```python
from build123d import *

# Parameters (mm, degrees)
SKETCH_1_R          = 28.5
SKETCH_1_W          = 5
SKETCH_1_H          = 57
EXTRUDE_1_DEPTH     = 5
SKETCH_2_R          = 1.6
SKETCH_2_R_2        = 20
EXTRUDE_2_DEPTH     = 5
FILLET_1_R          = 10
FILLET_2_R          = 5
SKETCH_3_R          = 1.6
SKETCH_3_R_2        = 7.5
CUT_EXTRUDE_1_DEPTH = 5


with BuildPart() as part:
    # 草图1 → 凸台-拉伸1 (new body)
    with BuildSketch(Plane(origin=(0, 0, 0), x_dir=(1, 0, 0), z_dir=(0, 1, 0))):
        with BuildLine():
            ThreePointArc((0, -28.5), (-28.5, 0), (0, 28.5))
            Line((0, 28.5), (-35, 28.5))
            Line((-35, 28.5), (-35, -28.5))
            Line((-35, -28.5), (0, -28.5))
        make_face()
        Circle(SKETCH_1_R)
        with Locations((-37.5, 0)):
            Rectangle(SKETCH_1_W, SKETCH_1_H)
    extrude(amount=EXTRUDE_1_DEPTH)

    # 草图2 → 凸台-拉伸2 (add)
    with BuildSketch(Plane.ZY.offset(40)):
        with BuildLine():
            Line((28.5, 0), (28.5, 40))
            ThreePointArc((28.5, 40), (0, 68.5), (-28.5, 40))
            Line((-28.5, 40), (-28.5, 0))
            Line((-28.5, 0), (28.5, 0))
        make_face()
        with Locations((12.5, 61.650635095)):
            Circle(SKETCH_2_R, mode=Mode.SUBTRACT)
        with Locations((-12.5, 18.349364905)):
            Circle(SKETCH_2_R, mode=Mode.SUBTRACT)
        with Locations((12.5, 18.349364905)):
            Circle(SKETCH_2_R, mode=Mode.SUBTRACT)
        with Locations((-25, 40)):
            Circle(SKETCH_2_R, mode=Mode.SUBTRACT)
        with Locations((-12.5, 61.650635095)):
            Circle(SKETCH_2_R, mode=Mode.SUBTRACT)
        with Locations((0, 40)):
            Circle(SKETCH_2_R_2, mode=Mode.SUBTRACT)
        with Locations((25, 40)):
            Circle(SKETCH_2_R, mode=Mode.SUBTRACT)
    extrude(amount=-EXTRUDE_2_DEPTH)

    # 圆角1
    fillet_1_edges = [part.edges().sort_by_distance(p)[0] for p in [
        (-40, 0, 0),
    ]]
    fillet(fillet_1_edges, radius=FILLET_1_R)

    # 圆角2
    fillet_2_edges = [part.edges().sort_by_distance(p)[0] for p in [
        (-35, 5, 0),
    ]]
    fillet(fillet_2_edges, radius=FILLET_2_R)

    # 草图3 → 切除-拉伸1 (cut)
    with BuildSketch(Plane(origin=(0, 5, 0), x_dir=(1, 0, 0), z_dir=(0, 1, 0))):
        with Locations((13.5, 0)):
            Circle(SKETCH_3_R)
        with Locations((6.75, -11.691342951)):
            Circle(SKETCH_3_R)
        with Locations((-6.75, -11.691342951)):
            Circle(SKETCH_3_R)
        with Locations((-13.5, 0)):
            Circle(SKETCH_3_R)
        with Locations((-6.75, 11.691342951)):
            Circle(SKETCH_3_R)
        with Locations((6.75, 11.691342951)):
            Circle(SKETCH_3_R)
        Circle(SKETCH_3_R_2)
    extrude(amount=-CUT_EXTRUDE_1_DEPTH, mode=Mode.SUBTRACT)


solid = part.part
```
For this review, take the finished solid that the model builds, in its own axes (mm). A direction names the side the tool comes from. Round coordinates to 2 decimals unless told otherwise and drop trailing zeros. Write each loop counter-clockwise with the first axis right and the second up, starting at its lowest first coordinate (ties: lowest second). Pieces come first, ordered by that corner, then holes. Notation, with made-up numbers: (54.25, -27.75) -> (109.25, -27.75) arc R16 ccw to (109.25, 3.25) -> close; hole circle Ø6 at (80.5, 37.5). An arc over 180 degrees is marked (long way). One line per question, with ' | ' between items. Start each with the question number.
(1) Add section B-B, the plane x = -13.5. Write out the cut boundary in (y, z).
(2) For line 1 along Z through (x, y) = (-6, 3); line 2 along Z through (x, y) = (-6.75, 2.85); line 3 along Y through (x, z) = (-26, 25.5), list the stretches that pass through material, from the lowest coordinate up. Write a range as from..to.
(3) Add section D-D, the plane z = 25. Write out the cut boundary in (x, y).
(4) Insertion check: P1, Ø3, axis at x = -13.5, z = 0, coming from the +Y side; P2, Ø2, axis at x = -31.5, z = 4, coming from the +Y side; P3, Ø8, axis at y = 36.5, z = 20.5, coming from the +X side; P4, Ø2, axis at x = 6, z = -8.5, coming from the +Y side. Each pin has a flat end and moves straight along its axis. Give the tip position at first contact, or say it passes through.
(5) Mouldability with a two-part tool opening along X and no side actions: class faces 1 (the face through (28.493, 2.465, 0.627)), 2 (the face through (6.542, 2.535, -13.278)), 3 (the face through (-8, 0, 0)) as released by +X, released by -X, zero draft, split by the parting line, or undercut.
(6) Add section A-A, the plane z = 0. Write out the cut boundary in (x, y).
(7) Tool access review of faces 4 (the face through (-35, 20, 6)), 5 (the face through (-40, 19, 0)): name each direction out of +Z, -Z, +X, -X, +Y, -Y from which nothing blocks a thin tool from reaching the whole face with its end or side.
(8) Add section C-C, the plane y = 23. Write out the cut boundary in (x, z).
Answer list:
1) outline: (0, -28.5) -> (5, -28.5) -> (5, -1.6) -> (0, -1.6) -> close; (0, 1.6) -> (5, 1.6) -> (5, 28.5) -> (0, 28.5) -> close
2) line 1: -28.5..-13.1, -10.28..-4.5, 4.5..10.28, 13.1..28.5 | line 2: -28.5..-13.29, -10.09..-3.27, 3.27..10.09, 13.29..28.5 | line 3: 0..5
3) outline: (-40, 10) arc R10 ccw to (-30, 0) -> (13.68, 0) -> (13.68, 5) -> (-30, 5) arc R5 cw to (-35, 10) -> (-35, 38.4) -> (-40, 38.4) -> close; (-40, 41.6) -> (-35, 41.6) -> (-35, 53.68) -> (-40, 53.68) -> close
4) P1: through | P2: y = 5.67 | P3: x = -35 | P4: y = 5
5) face 1: released by +X | face 2: undercut | face 3: zero draft
6) outline: (-40, 10) arc R10 ccw to (-30, 0) -> (-15.1, 0) -> (-15.1, 5) -> (-30, 5) arc R5 cw to (-35, 10) -> (-35, 20) -> (-40, 20) -> close; (-40, 60) -> (-35, 60) -> (-35, 68.5) -> (-40, 68.5) -> close; (-11.9, 0) -> (-7.5, 0) -> (-7.5, 5) -> (-11.9, 5) -> close; (7.5, 0) -> (11.9, 0) -> (11.9, 5) -> (7.5, 5) -> close; (15.1, 0) -> (28.5, 0) -> (28.5, 5) -> (15.1, 5) -> close
7) face 4: +Z, -Z, +X, +Y | face 5: +Z, -Z, -X, +Y, -Y
8) outline: (-40, -28.5) -> (-35, -28.5) -> (-35, -10.54) -> (-40, -10.54) -> close; (-40, 10.54) -> (-35, 10.54) -> (-35, 28.5) -> (-40, 28.5) -> close
